```python
from build123d import *

# Parameters (mm, degrees)
CUT_EXTRUDE1_DEPTH = 2.75
CHAMFER1_SIZE      = 0.5
CHAMFER2_SIZE      = 0.5


with BuildPart() as part:
    # Sketch1 → Revolve1 (revolve)
    with BuildSketch(Plane.XY, mode=Mode.PRIVATE) as revolve1_sk:
        Polygon((0, 0), (0, 4.75), (3, 4.75), (3, 2.5), (9, 2.5), (9, 0), align=None)
    revolve(revolve1_sk.sketch.rotate(Axis((9, 0, 0), (-1, 0, 0)), 90), axis=Axis((9, 0, 0), (-1, 0, 0)))

    # Sketch2 → Cut-Extrude1 (cut)
    with BuildSketch(Plane.ZY):
        Polygon((0, 2.309401077), (-2, 1.154700538), (-2, -1.154700538), (0, -2.309401077), (2, -1.154700538), (2, 1.154700538), align=None)
    extrude(amount=-CUT_EXTRUDE1_DEPTH, mode=Mode.SUBTRACT)

    # Chamfer1
    chamfer1_edges = [part.edges().sort_by_distance(p)[0] for p in [
        (9, 0, 2.5),
    ]]
    chamfer(chamfer1_edges, length=CHAMFER1_SIZE)

    # Chamfer2
    chamfer2_edges = [part.edges().sort_by_distance(p)[0] for p in [
        (0, 0, 4.75),
    ]]
    chamfer(chamfer2_edges, length=CHAMFER2_SIZE)


solid = part.part
```
Read the model definition and answer for the solid it produces. Units are mm, in the model's axes. A direction names the side the tool comes from. Give positions to 0.01 mm unless a question says otherwise; leave off trailing zeros. Write each loop counter-clockwise with the first axis right and the second up, starting at its lowest first coordinate (ties: lowest second). Pieces come first, ordered by that corner, then holes. Notation, with made-up numbers: (-34.5, 42) -> (-12.5, 42) arc R17 ccw to (-12.5, 53) -> close; hole circle Ø7 at (72, 52). An arc over 180 degrees is marked (long way). Answer in a Markdown table with one row per item.
1) Determine the mould class of faces 4 (the flat face through (2.75, 0, 0)), 5 (the cylindrical face through (1.768, 4.637, 1.03)), 6 (the flat face through (3, 2, -2)), 7 (the flat face through (1, 0, 2)) for opening direction Y: released by +Y, released by -Y, zero draft, split by the parting line, or undercut.
Results list:
| item | result |
|---|---|
| face 4 | undercut |
| face 5 | split by the parting line |
| face 6 | zero draft |
| face 7 | undercut |
2) Section B-B on y = 0 is taken. Give the vertices of the cut face in (x, z), plus the area to 3 significant figures.
Results list:
| item | result |
|---|---|
| outline | (0, -4.25) -> (0.5, -4.75) -> (3, -4.75) -> (3, -2.5) -> (8.5, -2.5) -> (9, -2) -> (9, 2) -> (8.5, 2.5) -> (3, 2.5) -> (3, 4.75) -> (0.5, 4.75) -> (0, 4.25) -> (0, 2) -> (2.75, 2) -> (2.75, -2) -> (0, -2) -> close |
| area | 47.0 mm^2 |
3) Section A-A on x = 2 is taken. Give the vertices of the cut face in (y, z), plus the area to 3 significant figures.
Results list:
| item | result |
|---|---|
| outline | circle Ø9.5 at (0, 0); hole (-2.31, 0) -> (-1.15, -2) -> (1.15, -2) -> (2.31, 0) -> (1.15, 2) -> (-1.15, 2) -> close |
| area | 57.0 mm^2 |
4) Each of these flat-tipped pins is pushed along its axis until it touches: pin 1 Ø2 at (x, y) = (5.5, -0.5) entering from -Z; pin 2 Ø4 at (x, z) = (7, 0.5) entering from -Y; pin 3 Ø1.5 at (x, z) = (6.5, 3) entering from +Y. Where does it stop, or does it pass through?
Results list:
| item | result |
|---|---|
| pin 1 | z = -2.5 |
| pin 2 | y = -2.5 |
| pin 3 | y = 1.09 |
5) Straight lines are drawn through the part: line 1 (X direction, y = 2.75, z = 0); line 2 (Y direction, x = 2, z = -1.75); line 3 (Y direction, x = 2, z = -0.25). For each, find the intervals that lie inside material, in ascending order. Write a range as [from, to].
Results list:
| item | result |
|---|---|
| line 1 | [0, 3] |
| line 2 | [-4.42, -1.3], [1.3, 4.42] |
| line 3 | [-4.74, -2.17], [2.17, 4.74] |
6) Section C-C on x = 3.5 is taken. Give the vertices of the cut face in (y, z), plus the area to 3 significant figures.
Results list:
| item | result |
|---|---|
| outline | circle Ø5 at (0, 0) |
| area | 19.6 mm^2 |
7) A tool of negligible diameter and unlimited length cuts with its end or side. For faces 1 (the flat face through (9, 0, 0)), 2 (the cylindrical face through (5.8, -0.1, 2.5)), 3 (the flat face through (1.36, -1.74, 0.99)), from which of +Z, -Z, +X, -X, +Y, -Y can it reach the whole face along a straight path? Write none if from no direction.
Results list:
| item | result |
|---|---|
| face 1 | +Z, -Z, +X, +Y, -Y |
| face 2 | +X |
| face 3 | -X |
